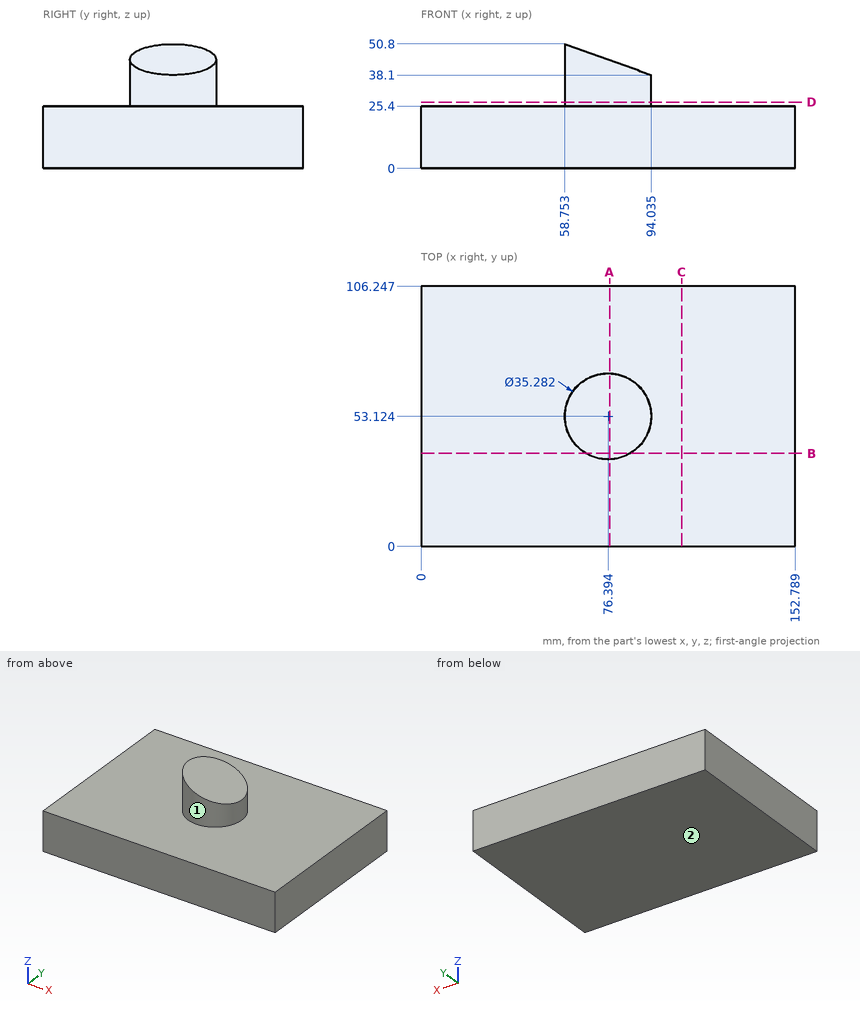
Could you check a few things on this drawing? It's one solid part, dimensions in mm from its lowest x, y, z. A direction names the side the tool comes from. Give positions to 0.01 mm unless a question says otherwise; leave off trailing zeros. Write each loop counter-clockwise with the first axis right and the second up, starting at its lowest first coordinate (ties: lowest second). Pieces come first, ordered by that corner, then holes. Notation, with made-up numbers: (8, 36) -> (32, 36) arc R27 cw to (32, 67) -> close; hole circle Ø5 at (75, 58). An arc over 180 degrees is marked (long way). Answer as CSV lines item,"result". Start each with the question number.
(1) Please list where these lines run through material, in increasing order: line 1 (Z direction, x = 139.5, y = 78.5); line 2 (X direction, y = 39, z = 26) (1 decimal).
(2) If we section it at C-C, the plane x = 106.5: Write out the boundary of the cut face in (y, z).
(3) If we section it at B-B, the plane y = 38: Write out the boundary of the cut face in (x, z) (1 decimal), and give its area (3 significant figures).
(4) I'm going to push flat-ended pins straight in: pin 1 Ø12 at (x, y) = (53, 57.5) entering from +Z; pin 2 Ø12 at (y, z) = (49, 34) entering from -X; pin 3 Ø6 at (x, z) = (72, 20) entering from -Y; pin 4 Ø10 at (x, y) = (82, 59.5) entering from +Z. Where does each tip first touch, or does it pass through?
(5) If we section it at D-D, the plane z = 27: Write out the boundary of the cut face in (x, y) (1 decimal), and give its area (3 significant figures).
(6) If we section it at A-A, the plane x = 77: Write out the boundary of the cut face in (y, z) (1 decimal).
(7) Which directions (+Z, -Z, +X, -X, +Y, -Y) give clear straight access to the entire face, cutting with the end or side of a thin tool? Please do the marked faces 1 and 2.
Answer list:
1,line 1,"0 to 25.4"
1,line 2,"65.8 to 87"
2,outline,"(0, 0) -> (106.25, 0) -> (106.25, 25.4) -> (0, 25.4) -> close"
3,outline,"(0, 0) -> (152.8, 0) -> (152.8, 25.4) -> (85.5, 25.4) -> (85.5, 41.2) -> (67.3, 47.7) -> (67.3, 25.4) -> (0, 25.4) -> close"
3,area,"4,230 mm^2"
4,pin 1,"z = 25.4"
4,pin 2,"x = 58.75"
4,pin 3,"y = 0"
4,pin 4,"z = 44.23"
5,outline,"circle Ø35.3 at (76.4, 53.1)"
5,area,"978 mm^2"
6,outline,"(0, 0) -> (106.2, 0) -> (106.2, 25.4) -> (70.8, 25.4) -> (70.8, 44.2) -> (35.5, 44.2) -> (35.5, 25.4) -> (0, 25.4) -> close"
7,face 1,"+Z"
7,face 2,"-Z, +X, -X, +Y, -Y"
